Input: part model. Units: mm. Frame: model coordinates. A direction names the side the tool comes from. Coordinates: 2 decimals unless noted, no trailing zeros. Write each loop counter-clockwise with the first axis right and the second up, starting at its lowest first coordinate (ties: lowest second). Pieces come first, ordered by that corner, then holes. Notation, with made-up numbers: M -13,58 L -7,58 A20 ccw -7,93 Z; hole C 73.25,-5 d1. An arc over 180 degrees is marked long. Write each question's results on one line, items separated by ' | '. Start each with the question number.
1. Section query D-D, the plane y = 19. Output: boundary loops of the cut face in (x, z), and give its area (3 significant figures).
2. Ray query, probe 1 along X at (y, z) = (27.55, 24.3); probe 2 along Z at (x, y) = (4.5, 38); probe 3 along Y at (x, z) = (-6.5, 21). Return the intervals inside material, ascending.
3. Pull-direction query (X, two-part tool) for faces 4 (the cylindrical face through (3.486, 27.914, 23.975)), 5 (the flat face through (0, 26.9, 24)), 6 (the flat face through (9.95, 23, 0)); classes: +X half, -X half, draft (parallel to the pull), parting line (faces both ways), or undercut.
4. Section query C-C, the plane x = 0. Output: boundary loops of the cut face in (y, z).
5. Set-up query: faces 1 (the flat face through (0, 37, -20.2)), 2 (the flat face through (0, 37, 20.2)), 3 (the flat face through (0, 13, 20.2)). Return all of +Z, -Z, +X, -X, +Y, -Y with unobstructed straight access to the full face (end or side cutting, diameter ignored); none if empty.
6. Section query A-A, the plane z = -24.3. Output: boundary loops of the cut face in (x, y), and give its area (3 significant figures).
7. First-contact query: pin 1 (2.5 mm diameter, centred on x = 0, z = -8, fed in from +Y); pin 2 (4 mm diameter, centred on x = -4.95, z = 24.3, fed in from +Y); pin 3 (10 mm diameter, centred on x = 4, y = 17, fed in from -Z). Flat tips, straight axial feed; report the tip coordinate or a pass-through.
8. Section query B-B, the plane x = -4.95. Output: boundary loops of the cut face in (y, z).
```python
from build123d import *

# Parameters (mm, degrees)
SKETCH_1_W          = 19.9
SKETCH_1_H          = 40.4
EXTRUDE_1_DEPTH     = 45.7
SKETCH_2_W          = 19.9
SKETCH_2_H          = 2
EXTRUDE_2_DEPTH     = 27
SKETCH_3_R          = 1.5
CUT_EXTRUDE_1_DEPTH = 3
SKETCH_5_R          = 1.5
CUT_EXTRUDE_2_DEPTH = 41.782502375


with BuildPart() as part:
    # 草图1 → 凸台-拉伸1 (new body)
    with BuildSketch(Plane(origin=(0, 0, 0), x_dir=(1, 0, 0), z_dir=(0, 1, 0))):
        Rectangle(SKETCH_1_W, SKETCH_1_H)
    extrude(amount=EXTRUDE_1_DEPTH)

    # 草图2 → 凸台-拉伸2 (add, symmetric)
    with BuildSketch(Plane.XY):
        with Locations((0, 27.9)):
            Rectangle(SKETCH_2_W, SKETCH_2_H)
    extrude(amount=EXTRUDE_2_DEPTH, both=True)

    # 草图3 → 切除-拉伸1 (cut)
    with BuildSketch(Plane(origin=(0, 45.7, 0), x_dir=(1, 0, 0), z_dir=(0, 1, 0))):
        with Locations(Location((0, 8, 0), (0, 0, 270))):
            Circle(SKETCH_3_R)
    extrude(amount=-CUT_EXTRUDE_1_DEPTH, mode=Mode.SUBTRACT)

    # 草图5 → 切除-拉伸2 (cut, through all)
    with BuildSketch(Plane(origin=(0, 28.9, 0), x_dir=(1, 0, 0), z_dir=(0, 1, 0))):
        with Locations(Location((-4.95, 24.3, 0), (0, 0, 270))):
            Circle(SKETCH_5_R)
        with Locations(Location((4.95, 24.3, 0), (0, 0, 270))):
            Circle(SKETCH_5_R)
        with Locations(Location((-4.95, -24.3, 0), (0, 0, 270))):
            Circle(SKETCH_5_R)
        with Locations(Location((4.95, -24.3, 0), (0, 0, 270))):
            Circle(SKETCH_5_R)
    extrude(amount=-CUT_EXTRUDE_2_DEPTH, mode=Mode.SUBTRACT)


solid = part.part
```
Answer:
1) outline: M -9.95,-20.2 L 9.95,-20.2 L 9.95,20.2 L -9.95,20.2 Z | area: 804 mm^2
2) probe 1: -9.95 to -6.45, -3.45 to 3.45, 6.45 to 9.95 | probe 2: -20.2 to 20.2 | probe 3: 26.9 to 28.9
3) face 4: undercut | face 5: draft | face 6: +X half
4) outline: M 0,-20.2 L 26.9,-20.2 L 26.9,-27 L 28.9,-27 L 28.9,-20.2 L 45.7,-20.2 L 45.7,-9.5 L 42.7,-9.5 L 42.7,-6.5 L 45.7,-6.5 L 45.7,20.2 L 28.9,20.2 L 28.9,27 L 26.9,27 L 26.9,20.2 L 0,20.2 Z
5) face 1: -Z, +X, -X, +Y | face 2: +Z, +X, -X, +Y | face 3: +Z, +X, -X, -Y
6) outline: M -9.95,26.9 L -6.45,26.9 L -6.45,28.9 L -9.95,28.9 Z; M -3.45,26.9 L 3.45,26.9 L 3.45,28.9 L -3.45,28.9 Z; M 6.45,26.9 L 9.95,26.9 L 9.95,28.9 L 6.45,28.9 Z | area: 27.8 mm^2
7) pin 1: y = 42.7 | pin 2: y = 28.9 | pin 3: z = -20.2
8) outline: M 0,-20.2 L 26.9,-20.2 L 26.9,-22.8 L 28.9,-22.8 L 28.9,-20.2 L 45.7,-20.2 L 45.7,20.2 L 28.9,20.2 L 28.9,22.8 L 26.9,22.8 L 26.9,20.2 L 0,20.2 Z; M 26.9,-27 L 28.9,-27 L 28.9,-25.8 L 26.9,-25.8 Z; M 26.9,25.8 L 28.9,25.8 L 28.9,27 L 26.9,27 Z
